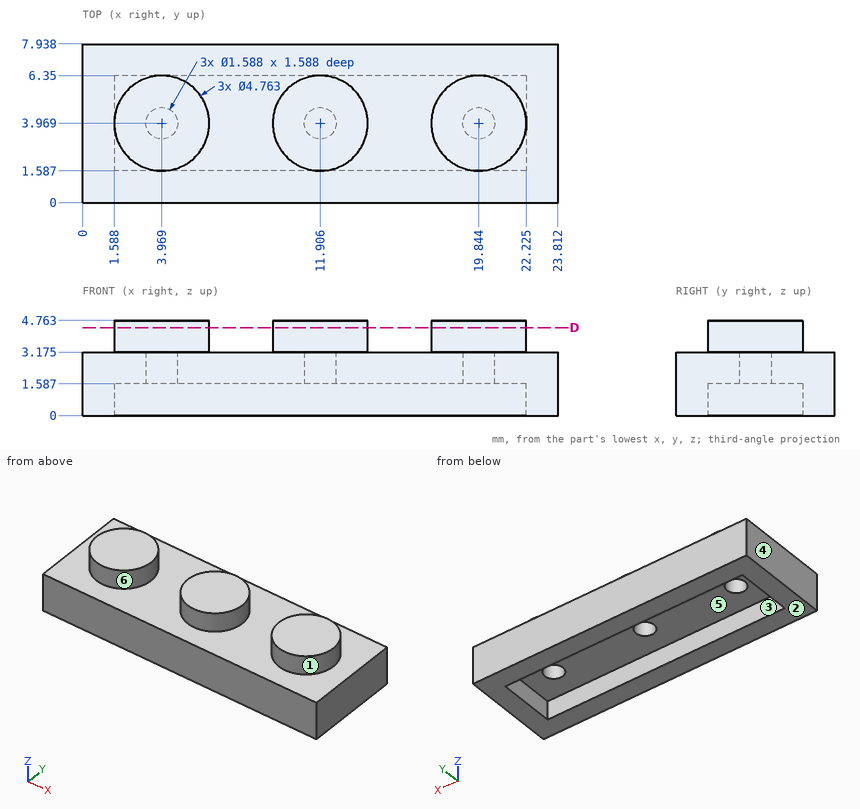
Source: three-view drawing plus pictorial views. Frame: mm from the lowest corner of the part. A direction names the side the tool comes from. Give positions to 0.01 mm unless a question says otherwise; leave off trailing zeros. Use CSV: the item, a comma, the result in double quotes.
(1) Pull-direction query (Y, two-part tool) for the marked faces 4, 5 and 6; classes: pulls with the +Y half, pulls with the -Y half, needs draft (parallel to the pull), parting line crosses it, or undercut.
Outcome:
face 4,"needs draft"
face 5,"undercut"
face 6,"parting line crosses it"
(2) Section D-D, the plane z = 4.4. Count the separate pieces of the cut face and the enclosed holes in it.
Outcome:
separate pieces,"3"
enclosed holes,"0"
(3) Pin query (flat end, axial travel): P1, Ø0.5, axis at x = 12, y = 4, coming from the -Z side (1 decimal); P2, Ø3, axis at x = 17.5, y = 5.5, coming from the -Z side; P3, Ø1.3, axis at x = 4, y = 3.5, coming from the -Z side. Return the tip coordinate at first contact, or that it passes through.
Outcome:
P1,"stops at z = 3.2"
P2,"stops at z = 0"
P3,"stops at z = 1.59"
(4) Material intervals for L1, parallel to X at y = 3.5, z = 0.8 (1 decimal); L2, parallel to X at y = 3, z = 4.45 (1 decimal); L3, parallel to Z at x = 21, y = 1 (1 decimal), sorted ascending. Write a range as [from, to].
Outcome:
L1,"x = [0, 1.6], [22.2, 23.8]"
L2,"x = [1.8, 6.1], [9.7, 14.1], [17.7, 22]"
L3,"z = [0, 3.2]"
(5) Set-up query: the marked faces 1, 2 and 3. Return all of +Z, -Z, +X, -X, +Y, -Y with unobstructed straight access to the full face (end or side cutting, diameter ignored); none if empty.
Outcome:
face 1,"+Z"
face 2,"-Z, +X, -X, +Y, -Y"
face 3,"-Z"
